```python
from build123d import *

# Parameters (mm, degrees)
ESQUISSE1_W             = 52
ESQUISSE1_H             = 44.3
BOSS_EXTRU_1_DEPTH      = 22.3
ESQUISSE4_W             = 38.9
ESQUISSE4_H             = 16.9
ENL_V_MAT_EXTRU_2_DEPTH = 52
BOSS_EXTRU_3_DEPTH      = 44.3
ENL_V_MAT_EXTRU_4_DEPTH = 38.9


with BuildPart() as part:
    # Esquisse1 → Boss.-Extru.1 (new body)
    with BuildSketch(Plane(origin=(0, 0, 0), x_dir=(1, 0, 0), z_dir=(0, 1, 0))):
        with Locations((-7.759163987, 0)):
            Rectangle(ESQUISSE1_W, ESQUISSE1_H)
    extrude(amount=BOSS_EXTRU_1_DEPTH)

    # Esquisse4 → Enlèv. mat.-Extru.2 (cut)
    with BuildSketch(Plane(origin=(18.240836013, 0, 0), x_dir=(0, 0, -1), z_dir=(1, 0, 0))):
        with Locations((0, 11.15)):
            Rectangle(ESQUISSE4_W, ESQUISSE4_H)
    extrude(amount=-ENL_V_MAT_EXTRU_2_DEPTH, mode=Mode.SUBTRACT)

    # Esquisse5 → Boss.-Extru.3 (add)
    with BuildSketch(Plane.XY.offset(22.15)):
        with BuildLine():
            Line((-33.759163987, 22.3), (-33.759163987, 0))
            ThreePointArc((-33.759163987, 0), (-44.909163987, 11.15), (-33.759163987, 22.3))
        make_face()
    extrude(amount=-BOSS_EXTRU_3_DEPTH)

    # Esquisse8 → Enlèv. mat.-Extru.4 (cut)
    with BuildSketch(Plane(origin=(0, 0, 19.45), x_dir=(-1, 0, 0), z_dir=(0, 0, -1))):
        with BuildLine():
            Line((33.759163987, 2.700004998), (33.759163987, 19.599995002))
            ThreePointArc((33.759163987, 19.599995002), (42.209158989, 11.15), (33.759163987, 2.700004998))
        make_face()
    extrude(amount=ENL_V_MAT_EXTRU_4_DEPTH, mode=Mode.SUBTRACT)


solid = part.part
```
Work out the finished part from the listing and answer in its coordinate system (mm). A direction names the side the tool comes from. Give positions to 0.01 mm unless a question says otherwise; leave off trailing zeros. Loops run counter-clockwise (first coordinate to the right, second up) from the corner with the lowest first, then second, coordinate; pieces in that order, holes last. Notation, with made-up numbers: (-5, 70) -> (44, 70) arc R23 ccw to (44, 79) -> close; hole circle Ø1 at (59, 83.25). An arc over 180 degrees is marked (long way). One line per question, with ' | ' between items. Start each with the question number.
1) Determine the mould class of faces 1 (the face through (-8, 0, 0)), 2 (the face through (-7, 19.6, 0)), 3 (the face through (-14, 11, 22.15)) for opening direction Y: +Y half, -Y half, draft (parallel to the pull), parting line (faces both ways), or undercut.
2) For faces 4 (the face through (-42.207, 11.336, 0.272)), 5 (the face through (-44.906, 10.905, 0.31)), determine the directions among +Z, -Z, +X, -X, +Y, -Y from which every point of the face is accessible in a straight line to the end or side of a thin tool.
3) Section A-A, the plane x = 2 is taken. Determine the outline of the cut face in (y, z).
4) Straight lines are drawn through the part: L1, parallel to Z at x = -20, y = 15.25; L2, parallel to Y at x = -30, z = -13.5. For each, find the intervals that lie inside material, in ascending order.
5) Each of these flat-tipped pins is pushed along its axis until it touches: pin 1 (1.5 mm diameter, centred on y = 15.5, z = -10, fed in from +X); pin 2 (1.5 mm diameter, centred on y = 3, z = -6.5, fed in from -X). Where does it stop, or does it pass through?
6) Section B-B, the plane y = 11.15 is taken. Determine the outline of the cut face in (x, z).
7) Section D-D, the plane y = 5.25 is taken. Determine the outline of the cut face in (x, z), then the cut area to 3 significant figures.
Resolved:
1) face 1: -Y half | face 2: undercut | face 3: draft
2) face 4: +X | face 5: +Z, -Z, -X
3) outline: (0, -22.15) -> (22.3, -22.15) -> (22.3, 22.15) -> (0, 22.15) -> close; hole (2.7, -19.45) -> (19.6, -19.45) -> (19.6, 19.45) -> (2.7, 19.45) -> close
4) L1: -22.15 to -19.45, 19.45 to 22.15 | L2: 0 to 2.7, 19.6 to 22.3
5) pin 1: x = -40.5 | pin 2: x = -42.1
6) outline: (-44.91, -22.15) -> (18.24, -22.15) -> (18.24, -19.45) -> (-42.21, -19.45) -> (-42.21, 19.45) -> (18.24, 19.45) -> (18.24, 22.15) -> (-44.91, 22.15) -> close
7) outline: (-43.22, -22.15) -> (18.24, -22.15) -> (18.24, -19.45) -> (-39.81, -19.45) -> (-39.81, 19.45) -> (18.24, 19.45) -> (18.24, 22.15) -> (-43.22, 22.15) -> close | area: 465 mm2
